The listing builds one solid part. Answer for the finished solid, in the listing's coordinates (mm). Face numbers are marked on the shaded views. A direction names the side the tool comes from. Give positions to 0.01 mm unless a question says otherwise; leave off trailing zeros. Order: outer loops, then holes, each group sorted by start corner. A loop starts at its lowest first (then second) coordinate and runs counter-clockwise, first axis right, second up. Notation, with made-up numbers: (24, 5) - (45, 5) arc R22 cw to (45, 24) - close; hole circle Ø8 at (-39.5, 43). An arc over 180 degrees is marked (long way). Answer as a JSON object with one key per item and string values. Group by question number.
Q1. A cutting plane is placed at B-B, the plane x = 32.5. Give the vertices of the cut face in (y, z).
Q2. For the marked faces 1 and 2, determine the directions among +Z, -Z, +X, -X, +Y, -Y from which every point of the face is accessible in a straight line to the end or side of a thin tool.
Q3. A cutting plane is placed at C-C, the plane z = -7.75. Count the separate pieces of the cut face and the enclosed holes in it, and give its area (3 significant figures).
Q4. The mould has two halves that part along X. Classify the marked faces 3, 4 and 5: released by +X, released by -X, zero draft, split by the parting line, or undercut.
Q5. A cutting plane is placed at A-A, the plane y = -45.5. Give the vertices of the cut face in (x, z).
Q6. Given pin 1 (10 mm diameter, centred on x = 11.5, y = -21, fed in from +Z); pin 2 (1.5 mm diameter, centred on y = -37, z = -5.5, fed in from -X); pin 3 (3 mm diameter, centred on y = -7, z = -2.5, fed in from +X); pin 4 (9 mm diameter, centred on y = -26, z = -7, fed in from +X), each flat-ended and moving along its own axis, determine where each tip first touches the part or whether it passes through.
Q7. Consider line 1 (Y direction, x = 0, z = -8.5); line 2 (X direction, y = -46, z = -9.75); line 3 (X direction, y = 0.5, z = -16.5). Determine where each line is inside the solid, lowest interval first.
from build123d import *

# Parameters (mm, degrees)
SKETCH_R          = 1.25
PAD_DEPTH         = 17.5
POCKET_DEPTH      = 53.501
POCKET_DEPTH_BACK = 0.001
POCKET001_DEPTH   = 5
PAD001_DEPTH      = 14.5
FILLET_R          = 1.99


with BuildPart() as part:
    # Sketch → Pad (new body)
    with BuildSketch(Plane.XY):
        with BuildLine():
            Line((0, 3.5), (67, 3.5))
            ThreePointArc((67, -3.5), (70.5, 0), (67, 3.5))
            ThreePointArc((67, -3.5), (64.87868, -4.37868), (64, -6.5))
            Line((64, -48), (64, -6.5))
            ThreePointArc((60, -48), (62, -50), (64, -48))
            Line((60, -48), (60, -7))
            ThreePointArc((60, -7), (58.974874, -4.525126), (56.5, -3.5))
            Line((56.5, -3.5), (10.5, -3.5))
            ThreePointArc((10.5, -3.5), (8.025126, -4.525126), (7, -7))
            Line((7, -7), (7, -48))
            ThreePointArc((3, -48), (5, -50), (7, -48))
            Line((3, -48), (3, -6.5))
            ThreePointArc((3, -6.5), (2.12132, -4.37868), (0, -3.5))
            ThreePointArc((0, 3.5), (-3.5, 0), (0, -3.5))
        make_face()
        Circle(SKETCH_R, mode=Mode.SUBTRACT)
        with Locations((67, 0)):
            Circle(SKETCH_R, mode=Mode.SUBTRACT)
    extrude(amount=-PAD_DEPTH)

    # Sketch001 (on Face4 of Pad) → Pocket (cut, two sides)
    with BuildSketch(Plane(origin=(0, 3.5, 0), x_dir=(-1, 0, 0), z_dir=(0, 1, 0))) as pocket_sk:
        with BuildLine():
            Line((-11, -17.5), (-52, -17.5))
            Line((-52, -17.5), (-52, -6.5))
            ThreePointArc((-48.5, -3), (-50.974874, -4.025126), (-52, -6.5))
            Line((-48.5, -3), (-14.5, -3))
            ThreePointArc((-11, -6.5), (-12.025126, -4.025126), (-14.5, -3))
            Line((-11, -6.5), (-11, -17.5))
        make_face()
        with BuildLine():
            Line((-56, -17.5), (-56, -6.5))
            ThreePointArc((-56, -6.5), (-57.025126, -4.025126), (-59.5, -3))
            Line((-59.5, -3), (-70.5, -3))
            Line((-70.5, -3), (-70.5, -17.5))
            Line((-70.5, -17.5), (-56, -17.5))
        make_face()
    extrude(amount=-POCKET_DEPTH, mode=Mode.SUBTRACT)
    extrude(pocket_sk.sketch, amount=POCKET_DEPTH_BACK, mode=Mode.SUBTRACT)

    # Sketch002 (on Face1 of Pocket) → Pocket001 (cut)
    with BuildSketch(Plane(origin=(3, 0, 0), x_dir=(0, -1, 0), z_dir=(-1, 0, 0))):
        with BuildLine():
            Line((7, 0), (7, -3.5))
            ThreePointArc((7, -3.5), (8.025126, -5.974874), (10.5, -7))
            Line((10.5, -7), (18.5, -7))
            ThreePointArc((18.5, -7), (20.974874, -5.974874), (22, -3.5))
            Line((22, -3.5), (22, 0))
            Line((22, 0), (7, 0))
        make_face()
    extrude(amount=-POCKET001_DEPTH, mode=Mode.SUBTRACT)

    # Sketch003 (on Face26 of Pocket001) → Pad001 (join)
    with BuildSketch(Plane(origin=(0, 0, -3), x_dir=(1, 0, 0), z_dir=(0, 0, -1))):
        with BuildLine():
            ThreePointArc((64, 48), (62, 50), (60, 48))
            Line((60, 48), (60, 43))
            ThreePointArc((60, 43), (62, 41), (64, 43))
            Line((64, 43), (64, 48))
        make_face()
    extrude(amount=PAD001_DEPTH)

    # Fillet
    fillet_edges = [part.edges().sort_by_distance(p)[0] for p in [
        (11, -3.5, -12),
        (11, 3.5, -12),
        (56, 3.5, -12),
        (52, 3.5, -12),
        (56, -3.5, -12),
        (52, -3.5, -12),
    ]]
    fillet(fillet_edges, radius=FILLET_R)


solid = part.part
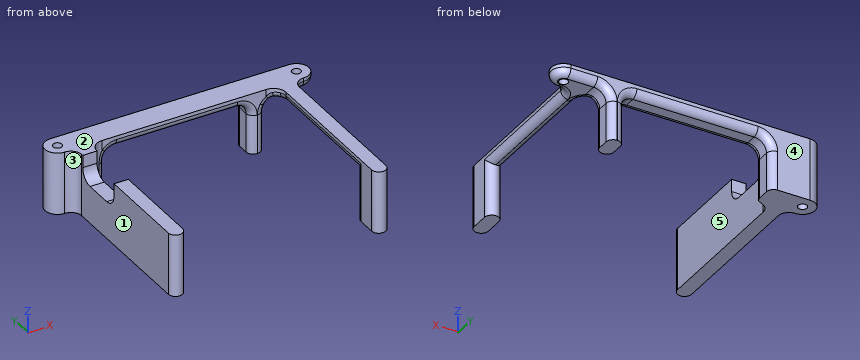
Reply:
{
 "1": {"outline": "(-3.5, -1.01) arc R1.99 ccw to (-1.51, -3) - (1.51, -3) arc R1.99 ccw to (3.5, -1.01) - (3.5, 0) - (-3.5, 0) - close"},
 "2": {"face 1": "+Z, -Z, -X, -Y", "face 2": "+Z, +X, -X, +Y, -Y"},
 "3": {"separate pieces": "3", "enclosed holes": "1", "area": "336 mm^2"},
 "4": {"face 3": "released by -X", "face 4": "zero draft", "face 5": "undercut"},
 "5": {"outline": "(3, -17.5) - (7, -17.5) - (7, 0) - (3, 0) - close; (60, -17.5) - (64, -17.5) - (64, 0) - (60, 0) - close"},
 "6": {"pin 1": "stops at z = 0", "pin 2": "stops at x = 3", "pin 3": "stops at x = 64.01", "pin 4": "stops at x = 63.33"},
 "7": {"line 1": "y = -3.5 to -1.25, 1.25 to 3.5", "line 2": "x = 3 to 7, 60 to 64", "line 3": "x = -3.46 to -1.15, 1.15 to 11, 52 to 56"}
}
